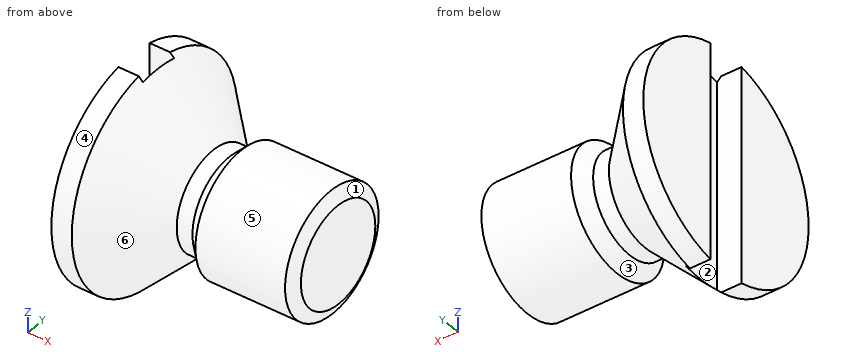
Autodesk Inventor part; units mm, degrees
ref_plane "Work Plane1" through (33.575, 0, 0) normal (0, 0, -1) x (1, 0, 0)
ref_plane "YZ Plane" through (0, 0, 0) normal (1, 0, 0) x (0, 1, 0)
ref_plane "XZ Plane" through (0, 0, 0) normal (0, 1, 0) x (-1, 0, 0)
sketch "Skizze1" plane through (0, 0, 0) normal (0, 0, 1) x (1, 0, 0)
  line L0 (0, 0) -> (5, 0)
  line L1 (5, 0) -> (5, 1.5)
  line L2 (5, 1.5) -> (2.65, 1.5)
  line L3 (2.65, 1.5) -> (2.3433, 1.1933)
  line L4 (2.3433, 1.1933) -> (1.9567, 1.1933)
  line L5 (1.9567, 1.1933) -> (0.5, 2.65)
  line L6 (0.5, 2.65) -> (0, 2.65)
  line L7 (0, 2.65) -> (0, 0)
  line L8 (2.65, 1.5) -> (1.65, 1.5) construction
  line L9 (-1, 0) -> (6, 0)
  line L10 (0, 3.18) -> (0, -0.53)
  dimension "d0" = 5
  dimension "d1" = 45
  dimension "d2" = 0.3067
  dimension "d3" = 2.35
  dimension "d4" = 1.65
  dimension "d5" = 2.3866
  dimension "d6" = 3
  dimension "d7" = 5.3
revolve "Körper" add sketch "Skizze1" angle 360 about axis through (0, 0, 0) along (1, 0, 0)
sketch "Skizze2" plane through (0, 0, 0) normal (-1, 0, 0) x (0, 0, 1)
  line L0 (2.65, -0.5) -> (-2.65, -0.5)
  line L1 (-2.65, -0.5) -> (-2.65, 0.5)
  line L2 (-2.65, 0.5) -> (2.65, 0.5)
  line L3 (2.65, 0.5) -> (2.65, -0.5)
  line L4 (0, 0.5) -> (0, -0.5) construction
  line L5 (-2.65, 0) -> (2.65, 0) construction
  line L6 (0, 2.65) -> (0, 0)
  dimension "d15" = 1
  dimension "d16" = 5.3
extrude "Loch" cut sketch "Skizze2" against normal blind 0.6
thread "Gewinde"
chamfer "Fase1" distance 0.3067 distance2 0.1534 1 edges at (5, -1.5, 0) measured on face at (5, 0.263, 0.1197)
ref_plane "Work Plane1" through (33.575, 0, 0) normal (0, 0, -1) x (1, 0, 0)
equation "\"d0\" = NLG"
equation "\"d1\" = 0.5 * SEWI"
equation "\"d2\" = GAL"
equation "\"d3\" = GEL"
equation "\"d4\" = KOH"
equation "\"d5\" = BDM"
equation "\"d6\" = GD"
equation "\"d7\" = KOD"
equation "\"d15\" = SBR"
equation "\"d16\" = KOD"
equation "\"d8\" = STI"
equation "\"d10\" = GEL"
equation "\"d12\" = -0.5 * SPD + 0.5 * GD"
equation "\"d13\" = 0.5 * GAL"
equation "\"NLG\" = 5"
equation "\"GAL\" = 0.61345 * PTC"
equation "\"GEL\" = 2.35"
equation "\"KOH\" = 1.65"
equation "\"KOD\" = 5.3"
equation "\"SEWI\" = 90deg"
equation "\"BDM\" = NND - 1.2269 * PTC"
equation "\"GD\" = NND"
equation "\"SBR\" = 1"
equation "\"STI\" = 0.6"
equation "\"SPD\" = NND - 1.2269 * PTC"
equation "\"GUL\" = 0.61345 * PTC"
equation "\"PTC\" = 0.5"
equation "\"EPV\" = 3.15"
equation "\"THREADDIA\" = 3"
equation "\"TOA\" = 30deg"
equation "\"RR\" = 0.3"
equation "\"NND\" = 3"
equation "\"GD1\" = THREADDIA - 1.2269 * PTC"
properties part number "AS 1427 - M3 x 5" material "Steel, Mild"
The model under review builds one solid part; all positions refer to its coordinate system, in mm. Face numbers are marked on the shaded views. A direction names the side the tool comes from. Round coordinates to 2 decimals unless told otherwise and drop trailing zeros. Write each loop counter-clockwise with the first axis right and the second up, starting at its lowest first coordinate (ties: lowest second). Pieces come first, ordered by that corner, then holes. Notation, with made-up numbers: M 73,66.25 L 114,66.25 A9 ccw 114,73.25 Z; hole C 8,27.5 d9. An arc over 180 degrees is marked long. Answer as CSV lines item,"result". Start each with the question number.
Q1. Consider section A-A, the plane y = 0. Give the boundary of the cut face in (x, z).
Q2. Wall thickness on line 1 along X through (y, z) = (0.65, -1.2); line 2 along X through (y, z) = (0.35, 1.1); line 3 along Z through (x, y) = (4.5, 0): over which ranges is each line inside the solid? List them lowest first.
Q3. Consider section C-C, the plane x = 1. Give the boundary of the cut face in (y, z), then the cut area to 3 significant figures.
Q4. Consider section D-D, the plane x = 4.6. Give the boundary of the cut face in (y, z), then the cut area to 3 significant figures.
Q5. Consider section B-B, the plane z = 0. Give the boundary of the cut face in (x, y), then the cut area to 3 significant figures.
Q6. Clearance check with flat-ended pins moving along their axes: P1, Ø3, axis at x = 4, z = 0.5, coming from the -Y side; P2, Ø0.5, axis at x = 0.5, z = 1.5, coming from the +Y side; P3, Ø3, axis at y = -1.5, z = 1.5, coming from the +X side; P4, Ø1, axis at x = 3, z = -1.5, coming from the -Y side. State where each tip first meets the part, or that it passes through.
Q7. Tool access review of the marked faces 4, 5 and 6: name each direction out of +Z, -Z, +X, -X, +Y, -Y from which nothing blocks a thin tool from reaching the whole face with its end or side.
Q8. The part is to be moulded in two halves that separate along X. For the marked faces 1, 2 and 3, say which applies: +X half, -X half, draft (parallel to the pull), parting line (faces both ways), or undercut.
Result set:
1,outline,"M 0.6,-2.55 L 1.96,-1.19 L 2.34,-1.19 L 2.65,-1.5 L 4.85,-1.5 L 5,-1.19 L 5,1.19 L 4.85,1.5 L 2.65,1.5 L 2.34,1.19 L 1.96,1.19 L 0.6,2.55 Z"
2,line 1,"x = 0 to 1.79, 2.51 to 4.91"
2,line 2,"x = 0.6 to 5"
2,line 3,"z = -1.5 to 1.5"
3,outline,"C 0,0 d4.3"
3,area,"14.5 mm²"
4,outline,"C 0,0 d3"
4,area,"7.07 mm²"
5,outline,"M 0,-2.65 L 0.5,-2.65 L 1.96,-1.19 L 2.34,-1.19 L 2.65,-1.5 L 4.85,-1.5 L 5,-1.19 L 5,1.19 L 4.85,1.5 L 2.65,1.5 L 2.34,1.19 L 1.96,1.19 L 0.5,2.65 L 0,2.65 L 0,0.5 L 0.6,0.5 L 0.6,-0.5 L 0,-0.5 Z"
5,area,"16.4 mm²"
6,P1,"stops at y = -1.5"
6,P2,"stops at y = 2.34"
6,P3,"stops at x = 5"
6,P4,"stops at y = -1.12"
7,face 4,"+X, -X, -Y"
7,face 5,"+X"
7,face 6,"none"
8,face 1,"+X half"
8,face 2,"-X half"
8,face 3,"undercut"
